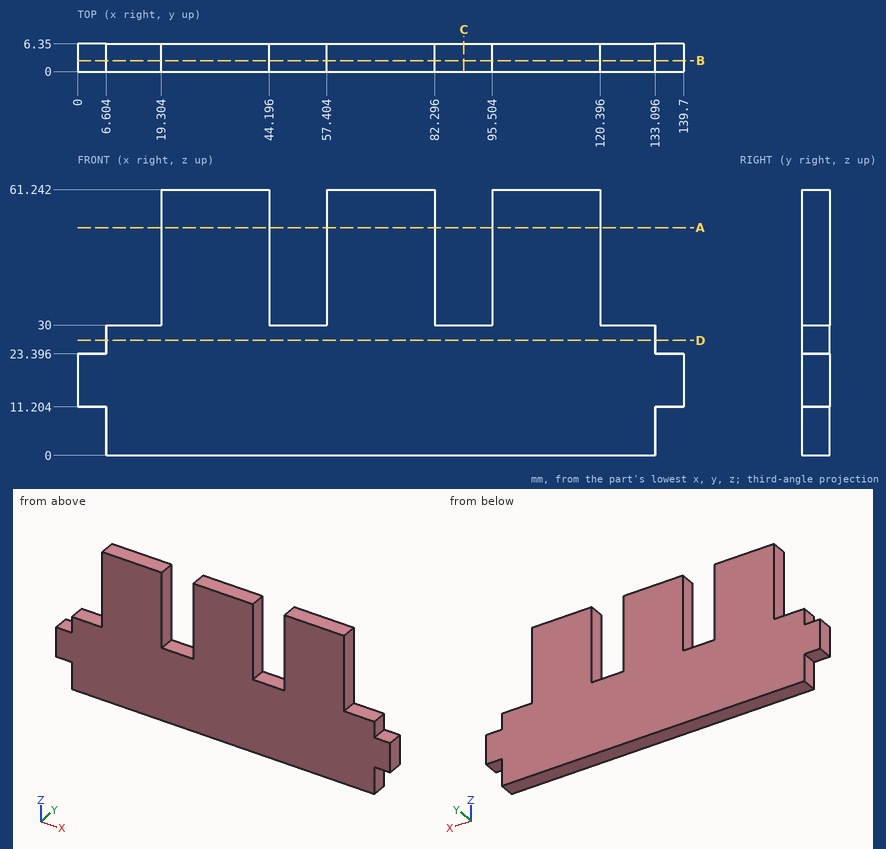
Drawing for the job (mm, zero at the part's lowest x, y, z). Coordinates: 2 decimals unless noted, no trailing zeros. Write each loop counter-clockwise with the first axis right and the second up, starting at its lowest first coordinate (ties: lowest second). Pieces come first, ordered by that corner, then holes. Notation, with made-up numbers: (59, -17.75) - (115, -17.75) arc R15 cw to (115, 10.25) - close; hole circle Ø3 at (70.5, 80). An arc over 180 degrees is marked (long way). Write each question's results on one line, items separated by ' | '. Start each with the question number.
1) Cut at D-D (z = 26.5). Write the cut outline in (x, y).
2) Flat gauge pins, fed straight in: P1, Ø3, axis at y = 2.5, z = 46, coming from the -X side; P2, Ø6, axis at x = 43.5, z = 20.5, coming from the -Y side; P3, Ø1.9, axis at y = 4.5, z = 3.5, coming from the +X side; P4, Ø1.9, axis at x = 2.5, y = 4, coming from the +Z side. Where does each tip first touch, or does it go through?
3) Cut at C-C (x = 89). Write the cut outline in (y, z), then the cut area to 4 significant figures.
4) Cut at A-A (z = 52.5). Write the cut outline in (x, y).
5) Cut at B-B (y = 2.5). Write the cut outline in (x, z), then the cut area to 3 significant figures.
6) Probe line 1 along X through (y, z) = (2.5, 55); line 2 along Z through (x, y) = (94, 4); line 3 along X through (y, z) = (2.5, 5). List the from-to ranges inside material, lowest first. Write a range as from..to.
Returned:
1) outline: (6.6, 0) - (133.1, 0) - (133.1, 6.35) - (6.6, 6.35) - close
2) P1: x = 19.3 | P2: y = 0 | P3: x = 133.1 | P4: z = 23.4
3) outline: (0, 0) - (6.35, 0) - (6.35, 30) - (0, 30) - close | area: 190.5 mm^2
4) outline: (19.3, 0) - (44.2, 0) - (44.2, 6.35) - (19.3, 6.35) - close; (57.4, 0) - (82.3, 0) - (82.3, 6.35) - (57.4, 6.35) - close; (95.5, 0) - (120.4, 0) - (120.4, 6.35) - (95.5, 6.35) - close
5) outline: (0, 11.2) - (6.6, 11.2) - (6.6, 0) - (133.1, 0) - (133.1, 11.2) - (139.7, 11.2) - (139.7, 23.4) - (133.1, 23.4) - (133.1, 30) - (120.4, 30) - (120.4, 61.24) - (95.5, 61.24) - (95.5, 30) - (82.3, 30) - (82.3, 61.24) - (57.4, 61.24) - (57.4, 30) - (44.2, 30) - (44.2, 61.24) - (19.3, 61.24) - (19.3, 30) - (6.6, 30) - (6.6, 23.4) - (0, 23.4) - close | area: 6,290 mm^2
6) line 1: 19.3..44.2, 57.4..82.3, 95.5..120.4 | line 2: 0..30 | line 3: 6.6..133.1
